```python
from build123d import *

# Parameters (mm, degrees)
F4_DEPTH        = 2.7018745767
F4_COPIES_COUNT = 3


# Not quite as in the source:
# - a pattern or mirror of a feature is missing from the dataset's text; its kind, count and spacing are read off the source's solid


with BuildPart() as f2:
    # F0 (on Front) → F2 (revolve)
    with BuildSketch(Plane.XZ):
        with BuildLine():
            Line((53.6962079262, 28.8167757166), (0, 28.8167757166))
            Line((0, 28.8167757166), (0, -215.1266485453))
            Line((0, -215.1266485453), (200, -215.1266485453))
            Line((200, -215.1266485453), (200, -212.5729433804))
            Line((200, -212.5729433804), (200, -207.1854621172))
            add(Edge.make_bspline(
                [(61.6075841476, 31.5186502934), (87.6578390598, -62.1243081987), (185.5585724115, -83.8800296187), (200, -207.1854621172)],
                knots=[0, 0, 0, 0, 275.9204850082, 275.9204850082, 275.9204850082, 275.9204850082], degree=3))
            Line((61.6075841476, 31.5186502934), (59, 31.5186502934))
            Line((59, 31.5186502934), (57, 31.5186502934))
            Line((57, 31.5186502934), (55, 31.5186502934))
            Line((55, 31.5186502934), (53.6962079262, 28.8167757166))
        make_face()
    revolve(axis=Axis((0, 0, -61.6418045454), (0, 0, -1)))

    # F3 (on face) → F4 (join, through all)
    with BuildSketch(Plane.XY.offset(31.5186502934)):
        Polygon((-1.5, 52.8230071068), (0, 52.8230071068), (1.5, 52.8230071068), (1.5, 55.3230071068), (0, 55.3230071068), (-1.5, 55.3230071068), align=None)
    f4 = extrude(amount=-F4_DEPTH)

    # F4_copies: F4 ×3 about axis
    f4_copies_axis = Axis((0, 0, 0), (0, 0, 1))
    for i in range(1, F4_COPIES_COUNT):
        add(f4.rotate(f4_copies_axis, i * 360 / F4_COPIES_COUNT))


solid = f2.part
```
Geometry: final body of the model. Coordinates: model frame, mm. A direction names the side the tool comes from. Coordinates: 2 decimals unless noted, no trailing zeros. Answer in a Markdown table with one row per item. Add a question column.
Q1. Line query: L1, parallel to Z at x = 38, y = -23.5; L2, parallel to X at y = 37, z = -195.5; L3, parallel to X at y = 105.5, z = -198. Output: solid intervals per line, ascending.
Q2. Contact query for flat-ended pins moving along their axis: P1, Ø4, axis at x = -109, z = -93.5, coming from the +Y side; P2, Ø3, axis at x = -18.5, z = -91.5, coming from the -Y side; P3, Ø1.5, axis at x = -13, z = -58.5, coming from the +Y side. Output: stop coordinate, or through.
Q3. Reachability of faces 4 (the flat face through (3, -3, -215.127)), 5 (the conical face through (-47.063, 26.283, 29.248)) from +Z, -Z, +X, -X, +Y, -Y: full face, straight path, thin tool, end or side. Return the list, or none.
Q4. Mould query, pull axis Y, two halves, no side actions, for faces 1 (the cylindrical face through (190.764, -60.075, -211.1)), 2 (the conical face through (46.29, 27.62, 29.25)), 3 (the flat face through (54.2, 11.2, 31.519)). Classes: released by +Y, released by -Y, zero draft, split by the parting line, or undercut.
Completed:
| question | item | result |
|---|---|---|
| 1 | L1 | z = -215.13 to 28.82 |
| 1 | L2 | x = -194.85 to 194.85 |
| 1 | L3 | x = -168.43 to 168.43 |
| 2 | P1 | stops at y = 105.91 |
| 2 | P2 | stops at y = -148.25 |
| 2 | P3 | stops at y = 118.37 |
| 3 | face 4 | -Z, +X, -X, +Y, -Y |
| 3 | face 5 | +Z |
| 4 | face 1 | split by the parting line |
| 4 | face 2 | undercut |
| 4 | face 3 | zero draft |
